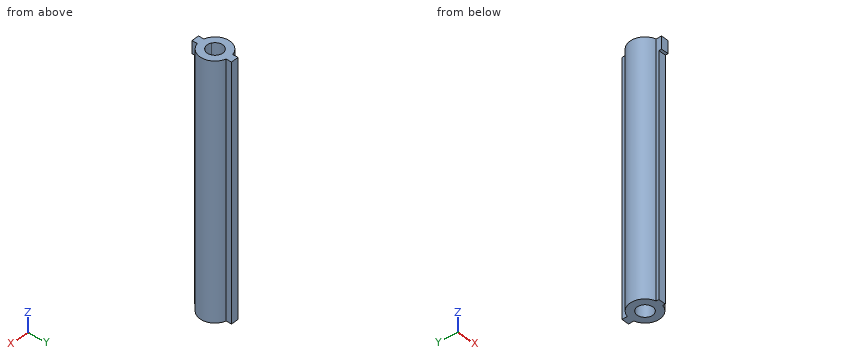
```python
from build123d import *

# Parameters (mm, degrees)
F0_R      = 7.62
F1_DEPTH  = 127
F2_R      = 3.96875
F3_DEPTH  = 19.05
F4_W      = 3.81
F4_H      = 20.32
F5_DEPTH  = 127
F7_DEPTH  = 19.05
F8_R      = 3.96875
F9_DEPTH  = 19.05
F10_W     = 3.81
F10_H     = 1.3909833627
F11_DEPTH = 120.65


with BuildPart() as f1:
    # F0 (on Top) → F1 (new body)
    with BuildSketch(Plane.XY):
        Circle(F0_R)
    extrude(amount=F1_DEPTH)

    # F2 (on face) → F3 (cut)
    with BuildSketch(Plane.XY.offset(127)):
        Circle(F2_R)
    extrude(amount=-F3_DEPTH, mode=Mode.SUBTRACT)

    # F4 (on Top) → F5 (join)
    with BuildSketch(Plane.XY):
        Rectangle(F4_W, F4_H)
    extrude(amount=F5_DEPTH)

    # F6 (on face) → F7 (cut)
    with BuildSketch(Plane.XY.offset(127)):
        with BuildLine():
            Line((1.905, -3.4816593117), (1.905, 3.4816593117))
            ThreePointArc((1.905, 3.4816593117), (0, 3.96875), (-1.905, 3.4816593117))
            Line((-1.905, 3.4816593117), (-1.905, -3.4816593117))
            ThreePointArc((-1.905, -3.4816593117), (0, -3.96875), (1.905, -3.4816593117))
        make_face()
    extrude(amount=-F7_DEPTH, mode=Mode.SUBTRACT)

    # F8 (on Top) → F9 (cut)
    with BuildSketch(Plane.XY):
        Circle(F8_R)
    extrude(amount=F9_DEPTH, mode=Mode.SUBTRACT)

    # F10 (on face) → F11 (cut)
    with BuildSketch(Plane(origin=(0, 0, 0), x_dir=(1, 0, 0), z_dir=(0, 0, -1))):
        with Locations((0, 9.4645083186)):
            Rectangle(F10_W, F10_H)
    extrude(amount=-F11_DEPTH, mode=Mode.SUBTRACT)


solid = f1.part
```
Model file for the job. Use its own axes, mm. Coordinates: 2 decimals unless noted, no trailing zeros. Order: outer loops, then holes, each group sorted by start corner. A loop starts at its lowest first (then second) coordinate and runs counter-clockwise, first axis right, second up. Notation, with made-up numbers: (13.5, -11) -> (62.5, -11) arc R19 ccw to (62.5, 9) -> close; hole circle Ø6 at (1.25, 79). An arc over 180 degrees is marked (long way). Answer as a JSON object with one key per item and string values. Group by question number.
1) Cut at A-A, the plane y = 0. Write the cut outline in (x, z).
2) Flat gauge pins, fed straight in: pin 1 (0.8 mm diameter, centred on y = -9.5, z = 47, fed in from -X); pin 2 (8.5 mm diameter, centred on x = 0, y = 0, fed in from +Z); pin 3 (0.8 mm diameter, centred on y = 8.5, z = 61, fed in from -X) (3 decimals); pin 4 (6.5 mm diameter, centred on x = 0, y = 0, fed in from +Z). Where does each tip first touch, or does it go through?
3) Cut at D-D, the plane x = 6. Write the cut outline in (y, z), then the cut area to 3 significant figures.
4) Cut at C-C, the plane z = 79. Write the cut outline in (x, y) (3 decimals).
5) Cut at B-B, the plane x = 0. Write the cut outline in (y, z).
6) Drill centre lines: L1, parallel to Y at x = 0, z = 14.5; L2, parallel to Y at x = -2, z = 74; L3, parallel to Z at x = 3.5, y = 1.75. Where is each one in solid material? Low to high.
Check values:
{
 "1": {"outline": "(-7.62, 0) -> (-3.97, 0) -> (-3.97, 19.05) -> (3.97, 19.05) -> (3.97, 0) -> (7.62, 0) -> (7.62, 127) -> (3.97, 127) -> (3.97, 107.95) -> (-3.97, 107.95) -> (-3.97, 127) -> (-7.62, 127) -> close"},
 "2": {"pin 1": "passes through", "pin 2": "stops at z = 127", "pin 3": "stops at x = -1.905", "pin 4": "stops at z = 107.95"},
 "3": {"outline": "(-4.7, 0) -> (4.7, 0) -> (4.7, 127) -> (-4.7, 127) -> close", "area": "1,190 mm²"},
 "4": {"outline": "(-1.905, -8.769) -> (1.905, -8.769) -> (1.905, -7.378) arc R7.62 ccw to (1.905, 7.378) -> (1.905, 10.16) -> (-1.905, 10.16) -> (-1.905, 7.378) arc R7.62 ccw to (-1.905, -7.378) -> close"},
 "5": {"outline": "(-10.16, 120.65) -> (-8.77, 120.65) -> (-8.77, 0) -> (-3.97, 0) -> (-3.97, 19.05) -> (3.97, 19.05) -> (3.97, 0) -> (10.16, 0) -> (10.16, 127) -> (3.97, 127) -> (3.97, 107.95) -> (-3.97, 107.95) -> (-3.97, 127) -> (-10.16, 127) -> close"},
 "6": {"L1": "y = -8.77 to -3.97, 3.97 to 10.16", "L2": "y = -7.35 to 7.35", "L3": "z = 19.05 to 107.95"}
}
